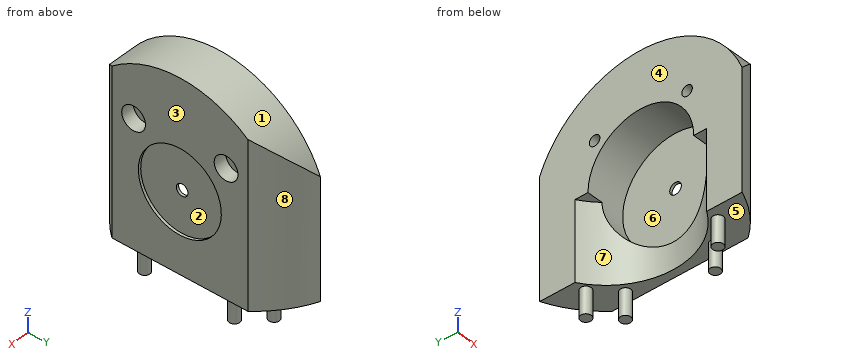
from build123d import *

# Parameters (mm, degrees)
SKETCH_1_W           = 17
SKETCH_1_H           = 82.4
EXTRUDE_1_DEPTH      = 30
EXTRUDE_2_DEPTH      = 17
CUT_EXTRUDE_1_DEPTH  = 62.2
SKETCH_4_R           = 2
EXTRUDE_3_DEPTH      = 10
SKETCH_5_R           = 20
CUT_EXTRUDE_2_DEPTH  = 15
SKETCH_6_R           = 15.7
CUT_EXTRUDE_3_DEPTH  = 1
SKETCH_7_R           = 2.2
CUT_EXTRUDE_4_DEPTH  = 1
SKETCH_8_R           = 29.2
CUT_EXTRUDE_7_DEPTH  = 30
SKETCH_9_R           = 4.5
CUT_EXTRUDE_9_DEPTH  = 5
SKETCH_10_R          = 2
CUT_EXTRUDE_10_DEPTH = 12


# Read off the part's stored shape, not the designer's step: 切除-拉伸1
with BuildPart() as part:
    # 草图1 → 凸台-拉伸1 (new body)
    with BuildSketch(Plane.XY):
        with Locations((23.7, 0)):
            Rectangle(SKETCH_1_W, SKETCH_1_H)
    extrude(amount=EXTRUDE_1_DEPTH)

    # 草图2 → 凸台-拉伸2 (add)
    with BuildSketch(Plane.ZY.offset(-15.2)):
        with BuildLine():
            Line((30, -41.2), (30, 41.2))
            ThreePointArc((30, 41.2), (71.2, 0), (30, -41.2))
        make_face()
    extrude(amount=-EXTRUDE_2_DEPTH)

    # 切除-拉伸1 outline → 切除-拉伸1 (cut)
    with BuildSketch(Plane.XY):
        with BuildLine():
            Line((32.2, -41.2), (32.2, -25.702139989))
            ThreePointArc((32.2, -25.702139989), (24.521954096, -33.107608904), (15.2, -38.293602599))
            Line((15.2, -38.293602599), (15.2, -41.2))
            Line((15.2, -41.2), (32.2, -41.2))
        make_face()
        with BuildLine():
            ThreePointArc((15.2, 38.293602599), (24.521954096, 33.107608904), (32.2, 25.702139989))
            Line((32.2, 25.702139989), (32.2, 41.2))
            Line((32.2, 41.2), (15.2, 41.2))
            Line((15.2, 41.2), (15.2, 38.293602599))
        make_face()
    extrude(amount=CUT_EXTRUDE_1_DEPTH, mode=Mode.SUBTRACT)

    # 草图4 → 凸台-拉伸3 (add)
    with BuildSketch(Plane.XY):
        with Locations((20, 25)):
            Circle(SKETCH_4_R)
        with Locations((28, 17)):
            Circle(SKETCH_4_R)
        with Locations((20, -25)):
            Circle(SKETCH_4_R)
        with Locations((28, -17)):
            Circle(SKETCH_4_R)
    extrude(amount=-EXTRUDE_3_DEPTH)

    # 草图5 → 切除-拉伸2 (cut)
    with BuildSketch(Plane.ZY.offset(-15.2)):
        with Locations(Location((30, 0, 0), (0, 0, 270))):
            Circle(SKETCH_5_R)
    extrude(amount=-CUT_EXTRUDE_2_DEPTH, mode=Mode.SUBTRACT)

    # 草图6 → 切除-拉伸3 (cut)
    with BuildSketch(Plane(origin=(32.2, 0, 0), x_dir=(0, 0, -1), z_dir=(1, 0, 0))):
        with Locations((-30, 0)):
            Circle(SKETCH_6_R)
    extrude(amount=-CUT_EXTRUDE_3_DEPTH, mode=Mode.SUBTRACT)

    # 草图7 → 切除-拉伸4 (cut)
    with BuildSketch(Plane(origin=(31.2, 0, 0), x_dir=(0, 0, -1), z_dir=(1, 0, 0))):
        with Locations((-30, 0)):
            Circle(SKETCH_7_R)
    extrude(amount=-CUT_EXTRUDE_4_DEPTH, mode=Mode.SUBTRACT)

    # 草图8 → 切除-拉伸7 (cut)
    with BuildSketch(Plane.XY):
        Circle(SKETCH_8_R)
    extrude(amount=CUT_EXTRUDE_7_DEPTH, mode=Mode.SUBTRACT)

    # 草图9 → 切除-拉伸9 (cut)
    with BuildSketch(Plane(origin=(32.2, 0, 0), x_dir=(0, 0, -1), z_dir=(1, 0, 0))):
        with Locations((-47.5, 17.5)):
            Circle(SKETCH_9_R)
        with Locations((-47.5, -17.5)):
            Circle(SKETCH_9_R)
    extrude(amount=-CUT_EXTRUDE_9_DEPTH, mode=Mode.SUBTRACT)

    # 草图10 → 切除-拉伸10 (cut)
    with BuildSketch(Plane(origin=(27.2, 0, 0), x_dir=(0, 0, -1), z_dir=(1, 0, 0))):
        with Locations((-47.5, 17.5)):
            Circle(SKETCH_10_R)
        with Locations((-47.5, -17.5)):
            Circle(SKETCH_10_R)
    extrude(amount=-CUT_EXTRUDE_10_DEPTH, mode=Mode.SUBTRACT)


solid = part.part
Work out the finished part from the listing and answer in its coordinate system (mm). Face numbers are marked on the shaded views. A direction names the side the tool comes from. Give positions to 0.01 mm unless a question says otherwise; leave off trailing zeros. Write each loop counter-clockwise with the first axis right and the second up, starting at its lowest first coordinate (ties: lowest second). Pieces come first, ordered by that corner, then holes. Notation, with made-up numbers: (23.25, 47) - (57.25, 47) arc R7 cw to (57.25, 60) - close; hole circle Ø3 at (-23.75, 28). An arc over 180 degrees is marked (long way). One line per item, written item: value. Start each with the question number.
1. For the marked faces 4, 5, 6, 7 and 8, determine the directions among +Z, -Z, +X, -X, +Y, -Y from which every point of the face is accessible in a straight line to the end or side of a thin tool.
2. Given pin 1 (25 mm diameter, centred on y = 0, z = 30, fed in from -X); pin 2 (1 mm diameter, centred on x = 23, z = 59, fed in from -Y); pin 3 (3 mm diameter, centred on x = 26.5, z = 25, fed in from +Y); pin 4 (3.5 mm diameter, centred on y = 0, z = 30, fed in from -X), each flat-ended and moving along its own axis, determine where each tip first touches the part or whether it passes through.
3. Consider probe 1 along Y at (x, z) = (28.35, 47.5); probe 2 along Y at (x, z) = (19, 47.5); probe 3 along X at (y, z) = (-4, 40). Determine where each line is inside the solid, lowest interval first.
4. Find section D-D (y = 6.5). Write down the section's boundary in (x, z), then the cut area to 3 significant figures.
5. Find section C-C (x = 20). Write down the section's boundary in (y, z), then the cut area to 3 significant figures.
6. Find section A-A (z = -4). Write down the section's boundary in (x, y).
7. For a pull along Y with two mould halves and no side action, classify the marked faces 1, 2 and 3 as +Y half, -Y half, draft (parallel to the pull), parting line (faces both ways), or undercut.
8. Find section B-B (z = 47.5). Write down the section's boundary in (x, y).
Geometry results:
1. face 4: +Z, -Z, -X, +Y, -Y
1. face 5: -Z
1. face 6: -X
1. face 7: -Z, -X
1. face 8: +Z, -Z, +X, +Y
2. pin 1: x = 30.2
2. pin 2: y = -29.75
2. pin 3: y = 32.75
2. pin 4: through
3. probe 1: -29.9 to -22, -13 to -9.68, 9.68 to 13, 22 to 29.9
3. probe 2: -36.56 to -19.5, -15.5 to -9.68, 9.68 to 15.5, 19.5 to 36.56
3. probe 3: 30.2 to 31.2
4. outline: (15.2, 48.91) - (30.2, 48.91) - (30.2, 11.09) - (28.47, 11.09) - (28.47, 0) - (32.2, 0) - (32.2, 15.71) - (31.2, 15.71) - (31.2, 44.29) - (32.2, 44.29) - (32.2, 70.68) - (15.2, 70.68) - close
4. area: 459 mm2
5. outline: (-36.02, 0) - (-27, 0) - (-27, -10) - (-23, -10) - (-23, 0) - (-21.28, 0) - (-21.28, 30) - (-20, 30) arc R20 cw to (20, 30) - (21.28, 30) - (21.28, 0) - (23, 0) - (23, -10) - (27, -10) - (27, 0) - (36.02, 0) - (36.02, 50) arc R41.2 ccw to (-36.02, 50) - close; hole circle Ø4 at (-17.5, 47.5); hole circle Ø4 at (17.5, 47.5)
5. area: 2,840 mm2
6. outline: circle Ø4 at (20, -25); circle Ø4 at (20, 25); circle Ø4 at (28, -17); circle Ø4 at (28, 17)
7. face 1: parting line
7. face 2: undercut
7. face 3: draft
8. outline: (15.2, -37.3) - (17.5, -37.3) arc R41.2 ccw to (32.2, -25.7) - (32.2, -22) - (27.2, -22) - (27.2, -19.5) - (15.2, -19.5) - close; (15.2, -15.5) - (27.2, -15.5) - (27.2, -13) - (32.2, -13) - (32.2, 13) - (27.2, 13) - (27.2, 15.5) - (15.2, 15.5) - (15.2, 9.68) - (30.2, 9.68) - (30.2, -9.68) - (15.2, -9.68) - close; (15.2, 19.5) - (27.2, 19.5) - (27.2, 22) - (32.2, 22) - (32.2, 25.7) arc R41.2 ccw to (17.5, 37.3) - (15.2, 37.3) - close
